Check sheet for the drawn part. Datum: minimum x, y, z corner. Units: mm. A direction names the side the tool comes from. Round coordinates to 2 decimals unless told otherwise and drop trailing zeros. Write each loop counter-clockwise with the first axis right and the second up, starting at its lowest first coordinate (ties: lowest second). Pieces come first, ordered by that corner, then holes.
Item 1: Go/stop test with flat-tipped pins: pin 1 Ø6.5 at (y, z) = (10, 29) entering from -X; pin 2 Ø2 at (x, y) = (11.5, 10) entering from +Z; pin 3 Ø1 at (x, y) = (52, 7) entering from +Z. Record where each tip stops, or that it passes through.
Item 2: Cross-section at C-C on z = 29. Enter the section's corners in (x, y), plus the area to 3 significant figures.
Item 3: Tool access check on the marked faces 1, 2, 3, 4 and 5. Record the directions out of +Z, -Z, +X, -X, +Y, -Y that give a thin tool (end or side, any length) a straight path to the whole face; none if there is none.
Item 4: Cross-section at A-A on y = 10. Enter the section's corners in (x, z).
Item 5: Material ranges on line 1 (Y direction, x = 5, z = 17); line 2 (Z direction, x = 16.15, y = 10); line 3 (Y direction, x = 55, z = 19.5), recorded low to high.
Item 6: Cross-section at B-B on y = 5. Enter the section's corners in (x, z).
Item 7: Cross-section at D-D on x = 5. Enter the section's corners in (y, z), plus the area to 3 significant figures.
Item 8: Release check for a two-part mould opening along Y. For the marked faces 6, 7 and 8 record: +Y half, -Y half, draft (parallel to the pull), parting line (faces both ways), or undercut.
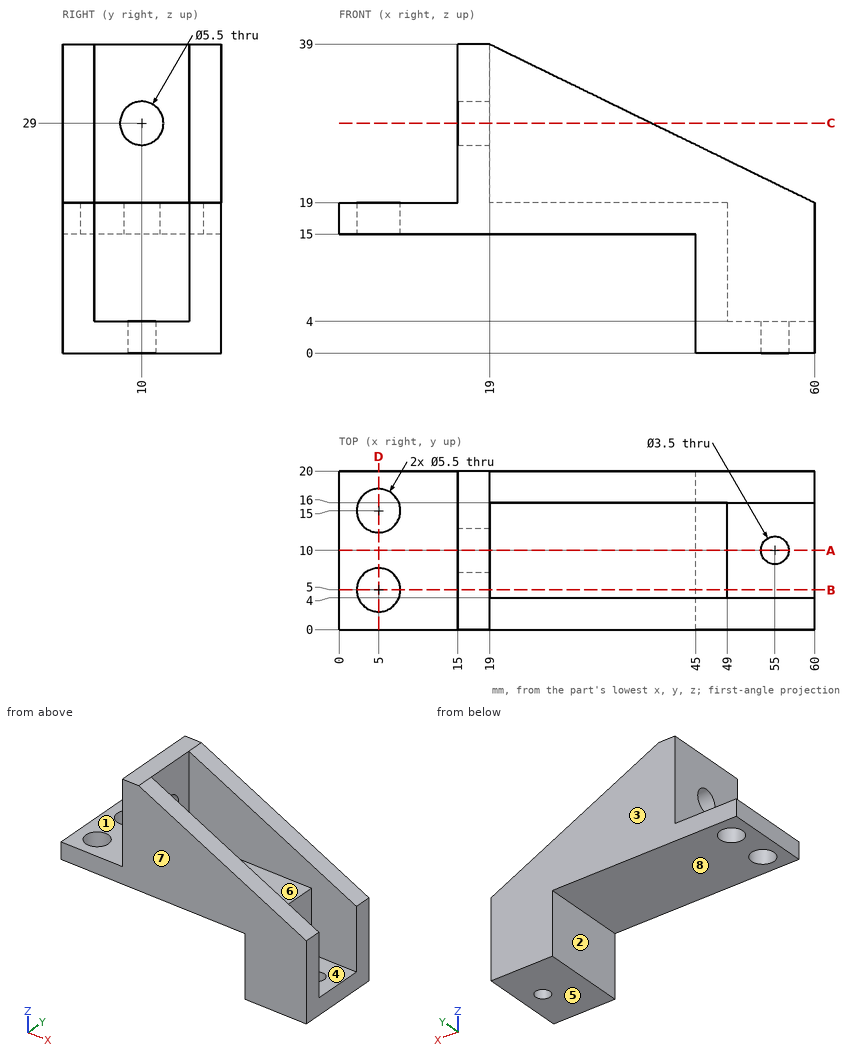
Response values:
1. pin 1: stops at x = 15
1. pin 2: stops at z = 19
1. pin 3: stops at z = 4
2. outline: (15, 0) - (39.5, 0) - (39.5, 4) - (19, 4) - (19, 7.25) - (15, 7.25) - close; (15, 12.75) - (19, 12.75) - (19, 16) - (39.5, 16) - (39.5, 20) - (15, 20) - close
2. area: 222 mm2
3. face 1: +Z, -X, +Y, -Y
3. face 2: -Z, -X, +Y, -Y
3. face 3: +Z, -Z, +X, -X, +Y
3. face 4: +Z, +X
3. face 5: -Z, +X, -X, +Y, -Y
4. outline: (0, 15) - (45, 15) - (45, 0) - (53.25, 0) - (53.25, 4) - (49, 4) - (49, 19) - (19, 19) - (19, 26.25) - (15, 26.25) - (15, 19) - (0, 19) - close; (15, 31.75) - (19, 31.75) - (19, 39) - (15, 39) - close; (56.75, 0) - (60, 0) - (60, 4) - (56.75, 4) - close
5. line 1: y = 0 to 2.25, 7.75 to 12.25, 17.75 to 20
5. line 2: z = 15 to 26.25, 31.75 to 39
5. line 3: y = 0 to 4, 16 to 20
6. outline: (0, 15) - (2.25, 15) - (2.25, 19) - (0, 19) - close; (7.75, 15) - (45, 15) - (45, 0) - (60, 0) - (60, 4) - (49, 4) - (49, 19) - (19, 19) - (19, 39) - (15, 39) - (15, 19) - (7.75, 19) - close
7. outline: (0, 15) - (2.25, 15) - (2.25, 19) - (0, 19) - close; (7.75, 15) - (12.25, 15) - (12.25, 19) - (7.75, 19) - close; (17.75, 15) - (20, 15) - (20, 19) - (17.75, 19) - close
7. area: 36.0 mm2
8. face 6: undercut
8. face 7: -Y half
8. face 8: draft
